```python
from build123d import *

# Parameters (mm, degrees)
F0_W        = 50.8
F0_H        = 101.6
F1_DEPTH    = 2
F2_T1_DEPTH = 127.7282991577
F2_T3_DEPTH = 76.9282991577
F3_W        = 15
F3_H        = 30
F3_W_2      = 16
F3_H_2      = 31
F3_R        = 8.5
F3_R_2      = 8
F3_R_3      = 7
F3_R_4      = 7.5
F3_R_5      = 2.5
F3_R_6      = 2
F3_R_7      = 1.5
F3_R_8      = 1
F3_R_9      = 0.5
F4_DEPTH    = 25.4


# Not quite as in the source:
# - a fillet or chamfer that OpenCascade refuses, or shapes differently, is made with other operations: its cross-section is extruded or revolved along the edge and cut away or added


with BuildPart() as f1:
    # F0 (on Top) → F1 (new body)
    with BuildSketch(Plane.XY):
        Rectangle(F0_W, F0_H)
    extrude(amount=F1_DEPTH)

    # F2: chamfer of 5.08 on 2 edges, made by hand

    # F2_s2 → F2_t1 (cut)
    with BuildSketch(Plane.XZ.offset(-63.8641495789)):
        Polygon((-25.4, -3.08), (-20.32, 2), (-25.4, 2), align=None)
    extrude(amount=F2_T1_DEPTH, mode=Mode.SUBTRACT)

    # F2_s4 → F2_t3 (cut)
    with BuildSketch(Plane.YZ.offset(-38.4641495789)):
        Polygon((50.8, -3.08), (45.72, 2), (50.8, 2), align=None)
    extrude(amount=F2_T3_DEPTH, mode=Mode.SUBTRACT)

    # F3 (on face) → F4 (cut)
    with BuildSketch(Plane.XY.offset(2)):
        with Locations((-7.5, -28.3660255373)):
            Rectangle(F3_W, F3_H)
        with Locations((13.9922183007, -27.6028160006)):
            Rectangle(F3_W_2, F3_H_2)
        with Locations((12.0123671368, 2.37495685)):
            Circle(F3_R)
        with Locations((-11.3166794181, 2.37495685)):
            Circle(F3_R_2)
        with Locations((-10.6418682262, 22.8119734675)):
            Circle(F3_R_3)
        with Locations((10.6627577916, 22.8119734675)):
            Circle(F3_R_4)
        with Locations((5.7463059202, 36.5009196103)):
            Circle(F3_R_5)
        with Locations((-0.1850809494, 36.5009196103)):
            Circle(F3_R_6)
        with Locations((-5.3699584678, 36.5009196103)):
            Circle(F3_R_7)
        with Locations((-9.3934237957, 36.5009196103)):
            Circle(F3_R_8)
        with Locations((-12.5698875636, 36.5009196103)):
            Circle(F3_R_9)
    extrude(amount=-F4_DEPTH, mode=Mode.SUBTRACT)


solid = f1.part
```
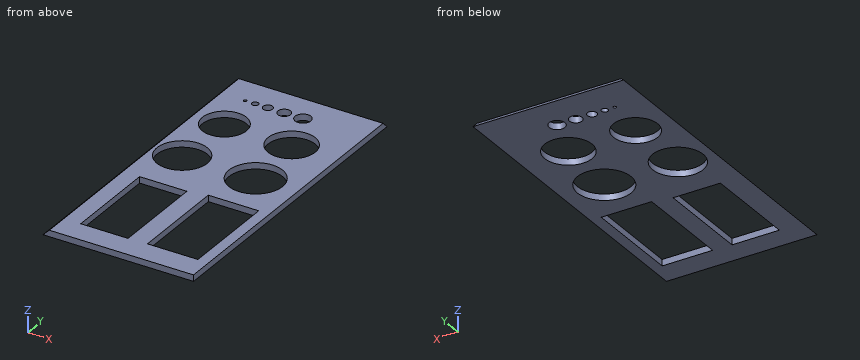
Part model, mm, in its own coordinate system. Coordinates: 2 decimals unless noted, no trailing zeros. Order: outer loops, then holes, each group sorted by start corner. A loop starts at its lowest first (then second) coordinate and runs counter-clockwise, first axis right, second up. Notation, with made-up numbers: (58.25, 86.25) -> (98.25, 86.25) arc R32 ccw to (98.25, 117.25) -> close; hole circle Ø7 at (20, -9.5). An arc over 180 degrees is marked (long way). Put each result on its own line as item: value. Start each with the question number.
(1) Band-saw the part on C-C (z = 1.6). Count the separate pieces of the cut face and the enclosed holes in it, then the cut area to 3 significant figures.
(2) Pin check, flat tips, straight feed: pin 1 Ø1.6 at (x, y) = (-9.39, 36.5) entering from +Z; pin 2 Ø1 at (x, z) = (-11, 1) entering from +Y; pin 3 Ø0.6 at (x, z) = (12, 1.5) entering from +Y. Stop position of each tip, or through.
(3) Band-saw the part on D-D (x = -5). Give the cut face in (y, z), then the cut area to 3 significant figures.
(4) Band-saw the part on B-B (x = 11). Give the cut face in (y, z), then the cut area to 3 significant figures.
(5) Band-saw the part on A-A (y = -29.5). Give the cut face in (x, z).
(6) Probe line 1 along X through (y, z) = (-33, 0.3); line 2 along X through (y, z) = (-2, 0.95); line 3 along Y through (x, z) = (11.5, 0.95). List the from-to ranges inside material, lowest first. Write a range as [from, to].
Determined:
1. separate pieces: 1
1. enclosed holes: 11
1. area: 2,720 mm²
2. pin 1: passes through
2. pin 2: stops at y = 47.22
2. pin 3: stops at y = 46.52
3. outline: (-50.8, 0) -> (-43.37, 0) -> (-43.37, 2) -> (-50.8, 2) -> close; (-13.37, 0) -> (-2.53, 0) -> (-2.53, 2) -> (-13.37, 2) -> close; (7.28, 0) -> (18.67, 0) -> (18.67, 2) -> (7.28, 2) -> close; (26.96, 0) -> (35.05, 0) -> (35.05, 2) -> (26.96, 2) -> close; (37.95, 0) -> (47.72, 0) -> (45.72, 2) -> (37.95, 2) -> close
3. area: 93.0 mm²
4. outline: (-50.8, 0) -> (-43.1, 0) -> (-43.1, 2) -> (-50.8, 2) -> close; (-12.1, 0) -> (-6.06, 0) -> (-6.06, 2) -> (-12.1, 2) -> close; (10.81, 0) -> (15.32, 0) -> (15.32, 2) -> (10.81, 2) -> close; (30.3, 0) -> (47.72, 0) -> (45.72, 2) -> (30.3, 2) -> close
4. area: 69.3 mm²
5. outline: (-22.32, 0) -> (-15, 0) -> (-15, 2) -> (-20.32, 2) -> close; (0, 0) -> (5.99, 0) -> (5.99, 2) -> (0, 2) -> close; (21.99, 0) -> (25.4, 0) -> (25.4, 2) -> (21.99, 2) -> close
6. line 1: x = [-22.02, -15], [0, 5.99], [21.99, 25.4]
6. line 2: x = [-21.37, -18.01], [-4.62, 4.72], [19.3, 25.4]
6. line 3: y = [-50.8, -43.1], [-12.1, -6.11], [10.86, 15.36], [30.27, 46.77]
